For this review, use the dimensioned drawing (mm, ordinates from the lowest corner) and the shaded views. A direction names the side the tool comes from. Give positions to 0.01 mm unless a question says otherwise; leave off trailing zeros. Write each loop counter-clockwise with the first axis right and the second up, starting at its lowest first coordinate (ties: lowest second). Pieces come first, ordered by that corner, then holes.
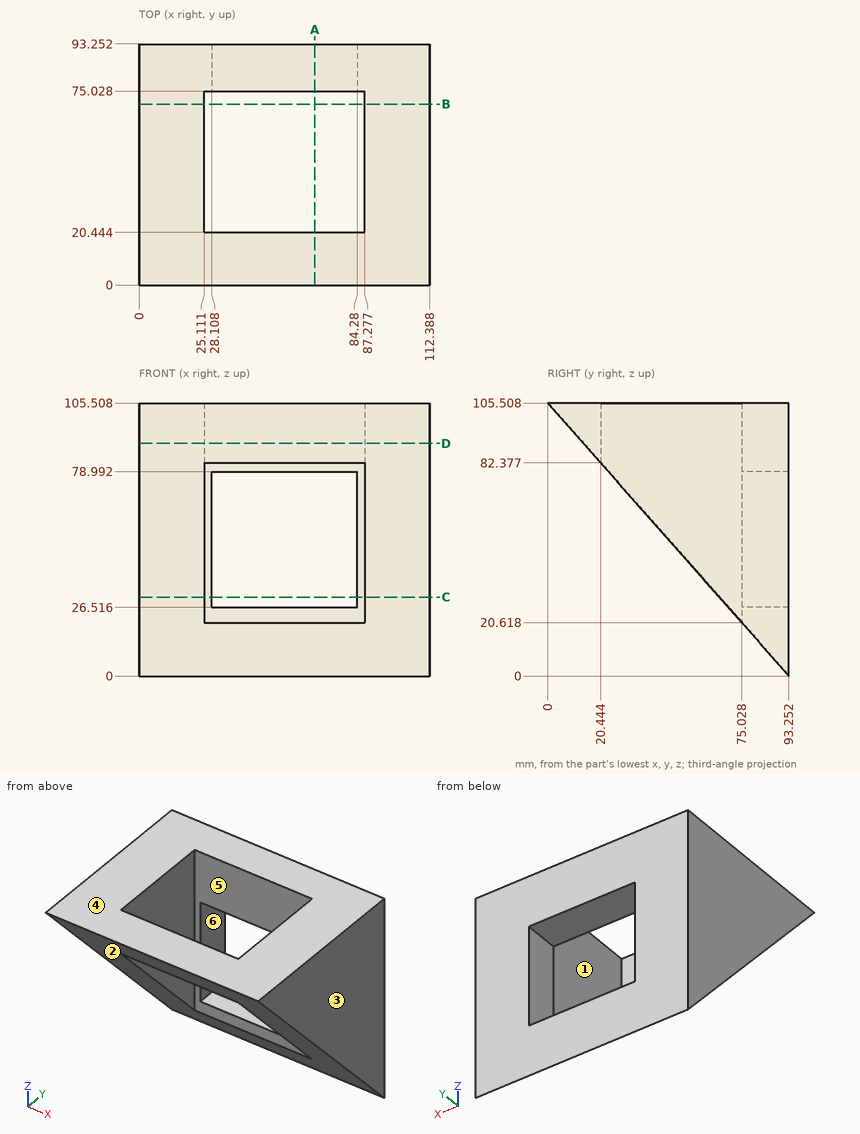
(1) The part is to be moulded in two halves that separate along X. For the marked faces 1, 2 and 3, say which applies: +X half, -X half, draft (parallel to the pull), parting line (faces both ways), or undercut.
(2) We need section D-D (z = 90). Write out the cut boundary in (x, y) (1 decimal).
(3) We need section C-C (z = 30.5). Write out the cut boundary in (x, y) (1 decimal), and give its area (3 significant figures).
(4) We need section B-B (y = 70). Write out the cut boundary in (x, z).
(5) For L1, parallel to X at y = 44.5, z = 81.5; L2, parallel to Y at x = 26.5, z = 30.5; L3, parallel to Y at x = 22, z = 86, list the stretches that pass through material, from the lowest coordinate up.
(6) Clearance check with flat-ended pins moving along their axes: pin 1 Ø5 at (x, y) = (13, 17) entering from -Z (1 decimal); pin 2 Ø5.5 at (x, y) = (43, 88) entering from -Z; pin 3 Ø10 at (x, y) = (21.5, 68) entering from -Z (1 decimal). State where each tip first meets the part, or that it passes through.
(7) Tool access review of the marked faces 4, 5 and 6: name each direction out of +Z, -Z, +X, -X, +Y, -Y from which nothing blocks a thin tool from reaching the whole face with its end or side.
(8) We need section A-A (x = 68). Write out the cut boundary in (y, z) (1 decimal), and give its area (4 significant figures).
The answers:
1. face 1: undercut
1. face 2: draft
1. face 3: +X half
2. outline: (0, 13.7) - (112.4, 13.7) - (112.4, 93.3) - (0, 93.3) - close; hole (25.1, 20.4) - (87.3, 20.4) - (87.3, 75) - (25.1, 75) - close
3. outline: (0, 66.3) - (25.1, 66.3) - (25.1, 75) - (28.1, 75) - (28.1, 93.3) - (0, 93.3) - close; (84.3, 75) - (87.3, 75) - (87.3, 66.3) - (112.4, 66.3) - (112.4, 93.3) - (84.3, 93.3) - close
3. area: 1,460 mm2
4. outline: (0, 26.31) - (25.11, 26.31) - (25.11, 105.51) - (0, 105.51) - close; (87.28, 26.31) - (112.39, 26.31) - (112.39, 105.51) - (87.28, 105.51) - close
5. L1: x = 0 to 25.11, 87.28 to 112.39
5. L2: y = 75.03 to 93.25
5. L3: y = 17.24 to 93.25
6. pin 1: stops at z = 83.4
6. pin 2: stops at z = 2.83
6. pin 3: stops at z = 22.9
7. face 4: +Z, +X, -X, +Y, -Y
7. face 5: +Z, -Z
7. face 6: +Y, -Y
8. outline: (0, 105.5) - (20.4, 82.4) - (20.4, 105.5) - close; (75, 20.6) - (93.3, 0) - (93.3, 26.5) - (75, 26.5) - close; (75, 79) - (93.3, 79) - (93.3, 105.5) - (75, 105.5) - close
8. area: 1,015 mm2
